Check sheet for the drawn part. Datum: minimum x, y, z corner. Units: mm. A direction names the side the tool comes from. Round coordinates to 2 decimals unless told otherwise and drop trailing zeros. Write each loop counter-clockwise with the first axis right and the second up, starting at its lowest first coordinate (ties: lowest second). Pieces come first, ordered by that corner, then holes. Notation, with made-up numbers: (70.25, -0.5) -> (120.25, -0.5) arc R17 ccw to (120.25, 8.5) -> close; hole circle Ø6 at (-27, 65). An arc over 180 degrees is marked (long way). Use a Markdown table: item, result.
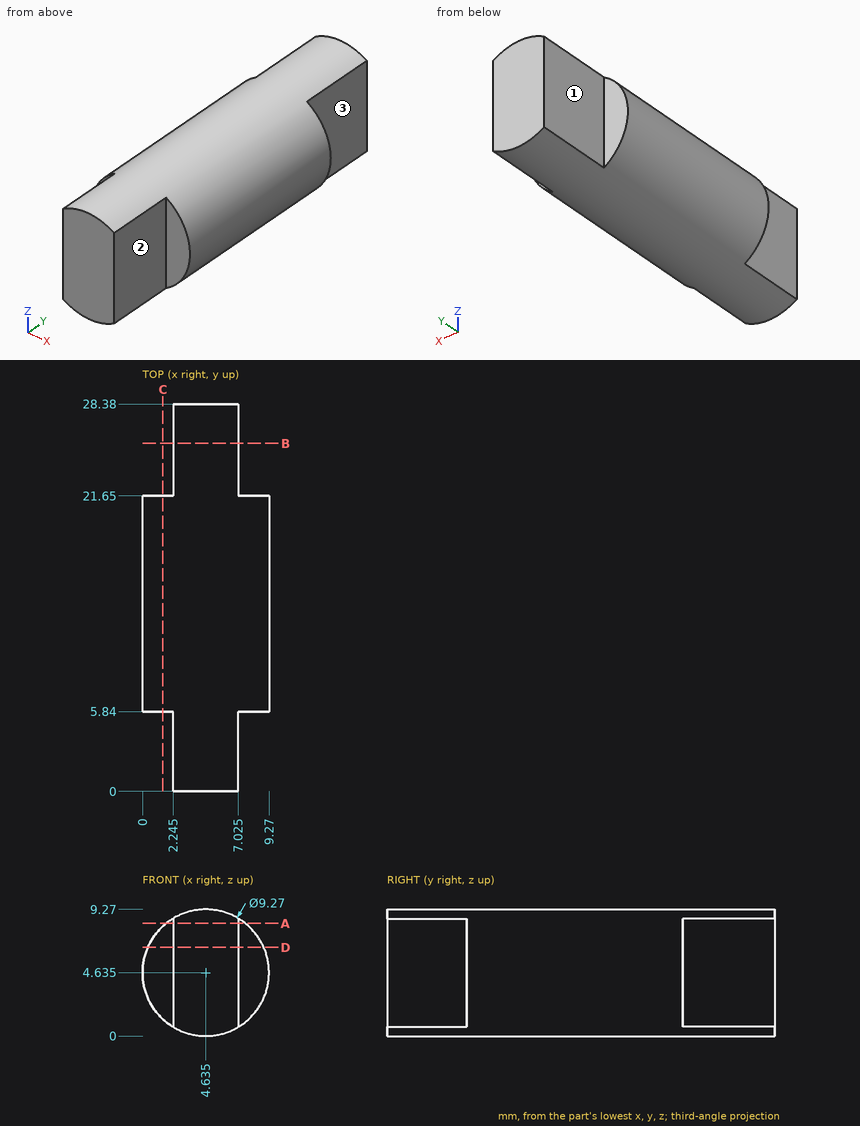
(1) Section check B-B on y = 25.5. Record the cut outline in (x, z) (3 decimals).
A:
| item | result |
|---|---|
| outline | (2.245, 0.664) arc R4.635 ccw to (7.025, 0.664) -> (7.025, 8.606) arc R4.635 ccw to (2.245, 8.606) -> close |
(2) Section check D-D on z = 6.5. Record the cut outline in (x, y) (3 decimals), plus the area to 3 significant figures.
A:
| item | result |
|---|---|
| outline | (0.392, 5.84) -> (2.245, 5.84) -> (2.245, 0) -> (7.025, 0) -> (7.025, 5.84) -> (8.878, 5.84) -> (8.878, 21.65) -> (7.025, 21.65) -> (7.025, 28.38) -> (2.245, 28.38) -> (2.245, 21.65) -> (0.392, 21.65) -> close |
| area | 194 mm2 |
(3) Section check C-C on x = 1.5. Record the cut outline in (y, z).
A:
| item | result |
|---|---|
| outline | (5.84, 1.22) -> (21.65, 1.22) -> (21.65, 8.05) -> (5.84, 8.05) -> close |
(4) Thickness scan on line 1 (Y direction, x = 1, z = 4.25); line 2 (X direction, y = 3.25, z = 2) (3 decimals); line 3 (Z direction, x = 4.5, y = 6.75). Record the ranges inside material, lowest first.
A:
| item | result |
|---|---|
| line 1 | y = 5.84 to 21.65 |
| line 2 | x = 2.245 to 7.025 |
| line 3 | z = 0 to 9.27 |
(5) Section check A-A on z = 8.25. Record the cut outline in (x, y) (3 decimals), plus the area to 3 significant figures.
A:
| item | result |
|---|---|
| outline | (1.734, 5.84) -> (2.245, 5.84) -> (2.245, 0) -> (7.025, 0) -> (7.025, 5.84) -> (7.536, 5.84) -> (7.536, 21.65) -> (7.025, 21.65) -> (7.025, 28.38) -> (2.245, 28.38) -> (2.245, 21.65) -> (1.734, 21.65) -> close |
| area | 152 mm2 |
(6) Access from +Z, -Z, +X, -X, +Y, -Y to the whole of each face (thin tool, end or side, straight path). Record for the marked faces 1, 2 and 3.
A:
| item | result |
|---|---|
| face 1 | +Z, -Z, -X, +Y |
| face 2 | +Z, -Z, +X, -Y |
| face 3 | +Z, -Z, +X, +Y |
(7) Gauge pin test, flat ends, axial feed: pin 1 Ø2 at (y, z) = (25, 6) entering from +X (3 decimals); pin 2 Ø5.5 at (y, z) = (26, 5.5) entering from -X (3 decimals); pin 3 Ø1 at (x, y) = (2.5, 7) entering from +Z; pin 4 Ø1.5 at (x, z) = (2, 4) entering from -Y. Record the tip position at first contact, or that the pin passes through.
A:
| item | result |
|---|---|
| pin 1 | stops at x = 7.025 |
| pin 2 | stops at x = 2.245 |
| pin 3 | stops at z = 8.97 |
| pin 4 | stops at y = 0 |
